from build123d import *

# Parameters (mm, degrees)
SKETCH1_R                = 88
BOSS_EXTRUDE3_DEPTH      = 25
SKETCH4_W                = 10.4719
SKETCH4_H                = 13.351164338
BOSS_EXTRUDE4_DEPTH      = 25
FILLET2_R                = 4
CIRPATTERN1_COUNT        = 30
FILLET2_OF_CIRPATTERN1_R = 4
SKETCH6_R                = 10
BOSS_EXTRUDE5_DEPTH      = 60
BOSS_EXTRUDE6_START      = 10
SKETCH7_R                = 10
BOSS_EXTRUDE6_DEPTH      = 10
SKETCH8_R                = 10
BOSS_EXTRUDE7_DEPTH      = 10
SKETCH9_R                = 10
BOSS_EXTRUDE8_DEPTH      = 25
SKETCH10_R               = 10
BOSS_EXTRUDE9_DEPTH      = 42.5
SKETCH12_R               = 12.5
CUT_EXTRUDE1_DEPTH       = 12
CUT_EXTRUDE2_START       = -55.5
SKETCH13_R               = 10
CUT_EXTRUDE2_DEPTH       = 55.5
SKETCH14_R               = 10
BOSS_EXTRUDE10_DEPTH     = 440
SKETCH15_R               = 105
BOSS_EXTRUDE12_DEPTH     = 25
BOSS_EXTRUDE13_START     = 30
SKETCH16_R               = 105
BOSS_EXTRUDE13_DEPTH     = 30
SKETCH17_R               = 10
BOSS_EXTRUDE14_DEPTH     = 50
SKETCH18_R               = 10
BOSS_EXTRUDE15_DEPTH     = 30
SKETCH19_R               = 105
SKETCH19_R_2             = 90
CUT_EXTRUDE3_DEPTH       = 100
SHELL3_START             = -30
SHELL3_OUTLINE_R         = 80
SHELL3_DEPTH             = 45


# Read off the part's stored shape, not the designer's step: Shell3
with BuildPart() as part:
    # Sketch1 → Boss-Extrude3 (new body)
    with BuildSketch(Plane.XY):
        Circle(SKETCH1_R)
    extrude(amount=BOSS_EXTRUDE3_DEPTH)

    # Sketch4 → Boss-Extrude4 (add)
    with BuildSketch(Plane.XY.offset(25)):
        with Locations((0, 93.324417831)):
            Rectangle(SKETCH4_W, SKETCH4_H)
    boss_extrude4 = extrude(amount=-BOSS_EXTRUDE4_DEPTH)

    # Fillet2
    fillet2_edges = [part.edges().sort_by_distance(p)[0] for p in [
        (5.23595, 100, 12.5),
        (0, 100, 0),
        (-5.23595, 100, 12.5),
        (0, 100, 25),
    ]]
    fillet(fillet2_edges, radius=FILLET2_R)

    # CirPattern1: Boss-Extrude4 ×30 about axis
    cirpattern1_axis = Axis((0, 0.317667884, 0), (0, 0, 1))
    for i in range(1, CIRPATTERN1_COUNT):
        add(boss_extrude4.rotate(cirpattern1_axis, i * 360 / CIRPATTERN1_COUNT))

    # Fillet2 of CirPattern1
    fillet2_of_cirpattern1_edges = [part.edges().sort_by_distance(p)[0] for p in [
        (-15.603590285, 98.910317096, 12.5),
        (-20.725122215, 97.821701879, 0),
        (-25.846654145, 96.733086661, 12.5),
        (-20.725122215, 97.821701879, 25),
        (-35.7611788, 93.511662322, 12.5),
        (-40.544457139, 91.382009596, 0),
        (-45.327735478, 89.252356869, 12.5),
        (-40.544457139, 91.382009596, 25),
        (-54.3558322, 84.039982796, 12.5),
        (-58.591804732, 80.962368605, 0),
        (-62.827777264, 77.884754413, 12.5),
        (-58.591804732, 80.962368605, 25),
        (-70.574874905, 70.909236365, 12.5),
        (-74.078409304, 67.018167216, 0),
        (-77.581943702, 63.127098067, 12.5),
        (-74.078409304, 67.018167216, 25),
        (-83.709456921, 54.693299655, 12.5),
        (-86.327431921, 50.158833942, 0),
        (-88.945406921, 45.624368229, 12.5),
        (-86.327431921, 50.158833942, 25),
        (-93.185533987, 36.100886913, 12.5),
        (-94.803531519, 31.121202547, 0),
        (-96.42152905, 26.14151818, 12.5),
        (-94.803531519, 31.121202547, 25),
        (-98.588956064, 15.944575793, 12.5),
        (-99.136261871, 10.737308875, 0),
        (-99.683567678, 5.530041957, 12.5),
        (-99.136261871, 10.737308875, 25),
        (-99.683567678, -4.894706189, 12.5),
        (-99.136261871, -10.101973107, 0),
        (-98.588956064, -15.309240025, 12.5),
        (-99.136261871, -10.101973107, 25),
        (-96.42152905, -25.506182413, 12.5),
        (-94.803531519, -30.485866779, 0),
        (-93.185533987, -35.465551145, 12.5),
        (-94.803531519, -30.485866779, 25),
        (-88.945406921, -44.989032461, 12.5),
        (-86.327431921, -49.523498174, 0),
        (-83.709456921, -54.057963887, 12.5),
        (-86.327431921, -49.523498174, 25),
        (-77.581943702, -62.491762299, 12.5),
        (-74.078409304, -66.382831448, 0),
        (-70.574874905, -70.273900597, 12.5),
        (-74.078409304, -66.382831448, 25),
        (-62.827777264, -77.249418645, 12.5),
        (-58.591804732, -80.327032837, 0),
        (-54.3558322, -83.404647029, 12.5),
        (-58.591804732, -80.327032837, 25),
        (-45.327735478, -88.617021102, 12.5),
        (-40.544457139, -90.746673828, 0),
        (-35.7611788, -92.876326554, 12.5),
        (-40.544457139, -90.746673828, 25),
        (-25.846654145, -96.097750894, 12.5),
        (-20.725122215, -97.186366111, 0),
        (-15.603590285, -98.274981329, 12.5),
        (-20.725122215, -97.186366111, 25),
        (-5.23595, -99.364664232, 12.5),
        (0, -99.364664232, 0),
        (5.23595, -99.364664232, 12.5),
        (0, -99.364664232, 25),
        (15.603590285, -98.274981329, 12.5),
        (20.725122215, -97.186366111, 0),
        (25.846654145, -96.097750894, 12.5),
        (20.725122215, -97.186366111, 25),
        (35.7611788, -92.876326554, 12.5),
        (40.544457139, -90.746673828, 0),
        (45.327735478, -88.617021102, 12.5),
        (40.544457139, -90.746673828, 25),
        (54.3558322, -83.404647029, 12.5),
        (58.591804732, -80.327032837, 0),
        (62.827777264, -77.249418645, 12.5),
        (58.591804732, -80.327032837, 25),
        (70.574874905, -70.273900597, 12.5),
        (74.078409304, -66.382831448, 0),
        (77.581943702, -62.491762299, 12.5),
        (74.078409304, -66.382831448, 25),
        (83.709456921, -54.057963887, 12.5),
        (86.327431921, -49.523498174, 0),
        (88.945406921, -44.989032461, 12.5),
        (86.327431921, -49.523498174, 25),
        (93.185533987, -35.465551145, 12.5),
        (94.803531519, -30.485866779, 0),
        (96.42152905, -25.506182413, 12.5),
        (94.803531519, -30.485866779, 25),
        (98.588956064, -15.309240025, 12.5),
        (99.136261871, -10.101973107, 0),
        (99.683567678, -4.894706189, 12.5),
        (99.136261871, -10.101973107, 25),
        (99.683567678, 5.530041957, 12.5),
        (99.136261871, 10.737308875, 0),
        (98.588956064, 15.944575793, 12.5),
        (99.136261871, 10.737308875, 25),
        (96.42152905, 26.14151818, 12.5),
        (94.803531519, 31.121202547, 0),
        (93.185533987, 36.100886913, 12.5),
        (94.803531519, 31.121202547, 25),
        (88.945406921, 45.624368229, 12.5),
        (86.327431921, 50.158833942, 0),
        (83.709456921, 54.693299655, 12.5),
        (86.327431921, 50.158833942, 25),
        (77.581943702, 63.127098067, 12.5),
        (74.078409304, 67.018167216, 0),
        (70.574874905, 70.909236365, 12.5),
        (74.078409304, 67.018167216, 25),
        (62.827777264, 77.884754413, 12.5),
        (58.591804732, 80.962368605, 0),
        (54.3558322, 84.039982796, 12.5),
        (58.591804732, 80.962368605, 25),
        (45.327735478, 89.252356869, 12.5),
        (40.544457139, 91.382009596, 0),
        (35.7611788, 93.511662322, 12.5),
        (40.544457139, 91.382009596, 25),
        (25.846654145, 96.733086661, 12.5),
        (20.725122215, 97.821701879, 0),
        (15.603590285, 98.910317096, 12.5),
        (20.725122215, 97.821701879, 25),
    ]]
    fillet(fillet2_of_cirpattern1_edges, radius=FILLET2_OF_CIRPATTERN1_R)

    # Sketch6 → Boss-Extrude5 (add)
    with BuildSketch(Plane.XY.offset(25)):
        Circle(SKETCH6_R)
    extrude(amount=BOSS_EXTRUDE5_DEPTH)

    # Sketch7 → Boss-Extrude6 (add)
    with BuildSketch(Plane(origin=(0, 0, 0), x_dir=(-1, 0, 0), z_dir=(0, 0, -1)).offset(BOSS_EXTRUDE6_START)):
        with Locations(Location((0, 0, 0), (0, 0, 180))):
            Circle(SKETCH7_R)
    extrude(amount=-BOSS_EXTRUDE6_DEPTH)

    # Sketch8 → Boss-Extrude7 (add)
    with BuildSketch(Plane.XY.offset(85)):
        Circle(SKETCH8_R)
    extrude(amount=BOSS_EXTRUDE7_DEPTH)

    # Sketch9 → Boss-Extrude8 (add)
    with BuildSketch(Plane.XY.offset(95)):
        Circle(SKETCH9_R)
    extrude(amount=BOSS_EXTRUDE8_DEPTH)

    # Sketch10 → Boss-Extrude9 (add)
    with BuildSketch(Plane.XY.offset(120)):
        Circle(SKETCH10_R)
    extrude(amount=BOSS_EXTRUDE9_DEPTH)

    # Sketch12 → Cut-Extrude1 (cut)
    with BuildSketch(Plane.XY.offset(162.5)):
        Circle(SKETCH12_R)
    extrude(amount=-CUT_EXTRUDE1_DEPTH, mode=Mode.SUBTRACT)

    # Sketch13 → Cut-Extrude2 (cut)
    with BuildSketch(Plane.XY.offset(150.5).offset(CUT_EXTRUDE2_START)):
        Circle(SKETCH13_R)
    extrude(amount=CUT_EXTRUDE2_DEPTH, mode=Mode.SUBTRACT)

    # Sketch14 → Boss-Extrude10 (add)
    with BuildSketch(Plane.XY.offset(95)):
        Circle(SKETCH14_R)
    extrude(amount=BOSS_EXTRUDE10_DEPTH)

    # Sketch15 → Boss-Extrude12 (add)
    with BuildSketch(Plane(origin=(0, 0, 0), x_dir=(-1, 0, 0), z_dir=(0, 0, -1))):
        Circle(SKETCH15_R)
    extrude(amount=-BOSS_EXTRUDE12_DEPTH)

    # Sketch16 → Boss-Extrude13 (add)
    with BuildSketch(Plane(origin=(0, 0, 0), x_dir=(-1, 0, 0), z_dir=(0, 0, -1)).offset(BOSS_EXTRUDE13_START)):
        Circle(SKETCH16_R)
    extrude(amount=-BOSS_EXTRUDE13_DEPTH)

    # Sketch17 → Boss-Extrude14 (add)
    with BuildSketch(Plane.XY.offset(535)):
        Circle(SKETCH17_R)
    extrude(amount=BOSS_EXTRUDE14_DEPTH)

    # Sketch18 → Boss-Extrude15 (add)
    with BuildSketch(Plane.XY.offset(585)):
        Circle(SKETCH18_R)
    extrude(amount=BOSS_EXTRUDE15_DEPTH)

    # Sketch19 → Cut-Extrude3 (cut)
    with BuildSketch(Plane(origin=(0, 0, -30), x_dir=(-1, 0, 0), z_dir=(0, 0, -1))):
        Circle(SKETCH19_R)
        Circle(SKETCH19_R_2, mode=Mode.SUBTRACT)
    extrude(amount=-CUT_EXTRUDE3_DEPTH, mode=Mode.SUBTRACT)

    # Shell3 outline → Shell3 (cut)
    with BuildSketch(Plane.XY.offset(SHELL3_START)):
        Circle(SHELL3_OUTLINE_R)
    extrude(amount=SHELL3_DEPTH, mode=Mode.SUBTRACT)


solid = part.part
Input: part model. Units: mm. Frame: model coordinates. A direction names the side the tool comes from. Round coordinates to 2 decimals unless told otherwise and drop trailing zeros. Write each loop counter-clockwise with the first axis right and the second up, starting at its lowest first coordinate (ties: lowest second). Pieces come first, ordered by that corner, then holes.
1) Draft query along Y for faces 4 (the cylindrical face through (-17.34, -78.1, -7.82)), 5 (the flat face through (60.4, -52.9, -30)), 6 (the cylindrical face through (-41.53, -79.845, -2.885)). Return one class per face: pulls with the +Y half, pulls with the -Y half, needs draft (parallel to the pull), parting line crosses it, or undercut.
2) Cut plane A-A (x = 0). Return the cut outline in (y, z), then the cut area to 3 significant figures.
3) Contact query for a flat-ended pin moving along its axis: P1, Ø12, axis at x = -9, y = 14.5, coming from the -Z side. Output: stop coordinate, or through.
4) Cut plane C-C (z = 356). Return the cut outline in (x, y).
5) Reachability of faces 1 (the flat face through (0, 0, 615)), 2 (the cylindrical face through (-2.17, -9.76, 315.87)), 3 (the flat face through (-1, 1, 15)) from +Z, -Z, +X, -X, +Y, -Y: full face, straight path, thin tool, end or side. Return the list, or none.
6) Ray query, L1, parallel to Y at x = 0, z = -12; L2, parallel to Z at x = -12.5, y = -51.5; L3, parallel to Z at x = 29, y = -83. Return the intervals inside material, ascending.
7) Cut plane D-D (y = -65.5). Return the cut outline in (x, z).
Geometry says:
1. face 4: undercut
1. face 5: needs draft
1. face 6: parting line crosses it
2. outline: (-90, -30) - (-80, -30) - (-80, 15) - (80, 15) - (80, -30) - (90, -30) - (90, 25) - (10, 25) - (10, 615) - (-10, 615) - (-10, 25) - (-90, 25) - close
2. area: 14,500 mm2
3. P1: stops at z = 15
4. outline: circle Ø20 at (0, 0)
5. face 1: +Z, +X, -X, +Y, -Y
5. face 2: +Z
5. face 3: -Z
6. L1: y = -90 to -80, 80 to 90
6. L2: z = 15 to 25
6. L3: z = -30 to 25
7. outline: (-61.72, -30) - (-45.93, -30) - (-45.93, 15) - (45.93, 15) - (45.93, -30) - (61.72, -30) - (61.72, 25) - (-61.72, 25) - close
